The listing builds one solid part. Answer for the finished solid, in the listing's coordinates (mm). A direction names the side the tool comes from. Coordinates: 2 decimals unless noted, no trailing zeros. Order: outer loops, then holes, each group sorted by start corner. A loop starts at its lowest first (then second) coordinate and runs counter-clockwise, first axis right, second up. Notation, with made-up numbers: (57, 7) -> (77, 7) arc R18 ccw to (77, 22) -> close; hole circle Ø8 at (60, -33). An arc over 180 degrees is marked (long way). Write each question's results on one line, items separated by ' | '. Start each with the question number.
(1) Determine the mould class of faces 4 (the face through (-30, 0, 15)), 5 (the face through (39.724, -14.852, 3.204)), 6 (the face through (0, 0, 24.5)) for opening direction X: +X half, -X half, draft (parallel to the pull), parting line (faces both ways), or undercut.
(2) Straight lines are drawn through the part: L1, parallel to X at y = -13.5, z = 3; L2, parallel to X at y = 14.5, z = 5.75; L3, parallel to Y at x = -38.25, z = 4.75. For each, find the intervals that lie inside material, in ascending order.
(3) The part is cut by section D-D, the plane y = -13.5. Give the vertices of the cut face in (x, z), then the cut area to 3 significant figures.
(4) The part is cut by section A-A, the plane z = 3.5. Give the vertices of the cut face in (x, y), then the cut area to 3 significant figures.
(5) A tool of negligible diameter and unlimited length cuts with its end or side. For faces 1 (the face through (-36, 0, 6.5)), 2 (the face through (39.724, 12.148, 3.204)), 3 (the face through (30, 0, 15)), from which of +Z, -Z, +X, -X, +Y, -Y can it reach the whole face along a straight path? Write none if from no direction.
(6) The part is cut by section B-B, the plane y = -4. Give the vertices of the cut face in (x, z), then the cut area to 3 significant figures.
(7) Given pin 1 (2 mm diameter, centred on y = 12, z = 16, fed in from -X); pin 2 (5 mm diameter, centred on y = -6.5, z = 14, fed in from +X); pin 3 (3.5 mm diameter, centred on x = -34.5, y = 5, fed in from +Z); pin 4 (2.5 mm diameter, centred on x = -38.25, y = -13.5, fed in from +Z), each flat-ended and moving along its own axis, determine where each tip first touches the part or whether it passes through.
(8) The part is cut by section C-C, the plane x = 38.25. Give the vertices of the cut face in (y, z), then the cut area to 3 significant figures.
```python
from build123d import *

# Parameters (mm, degrees)
SKETCH_1_R      = 2
EXTRUDE_1_DEPTH = 6.5
SKETCH_2_W      = 60
SKETCH_2_H      = 40
EXTRUDE_2_DEPTH = 18


with BuildPart() as part:
    # ｽｹｯﾁ1 → ﾎﾞｽ - 押し出し1 (new body)
    with BuildSketch(Plane.XY):
        with BuildLine():
            Line((33, -20), (-33, -20))
            ThreePointArc((-33, -20), (-39.363961031, -17.363961031), (-42, -11))
            Line((-42, -11), (-42, 11))
            ThreePointArc((-42, 11), (-39.363961031, 17.363961031), (-33, 20))
            Line((-33, 20), (33, 20))
            ThreePointArc((33, 20), (39.363961031, 17.363961031), (42, 11))
            Line((42, 11), (42, -11))
            ThreePointArc((42, -11), (39.363961031, -17.363961031), (33, -20))
        make_face()
        with Locations(Location((-38.25, 13.5, 0), (0, 0, 180))):
            Circle(SKETCH_1_R, mode=Mode.SUBTRACT)
        with Locations(Location((38.25, 13.5, 0), (0, 0, 180))):
            Circle(SKETCH_1_R, mode=Mode.SUBTRACT)
        with Locations(Location((38.25, -13.5, 0), (0, 0, 180))):
            Circle(SKETCH_1_R, mode=Mode.SUBTRACT)
        with Locations(Location((-38.25, -13.5, 0), (0, 0, 180))):
            Circle(SKETCH_1_R, mode=Mode.SUBTRACT)
    extrude(amount=EXTRUDE_1_DEPTH)

    # ｽｹｯﾁ2 → ﾎﾞｽ - 押し出し2 (add)
    with BuildSketch(Plane.XY.offset(6.5)):
        Rectangle(SKETCH_2_W, SKETCH_2_H)
    extrude(amount=EXTRUDE_2_DEPTH)


solid = part.part
```
Established:
1) face 4: -X half | face 5: undercut | face 6: draft
2) L1: x = -41.65 to -40.25, -36.25 to 36.25, 40.25 to 41.65 | L2: x = -41.29 to -39.98, -36.52 to 36.52, 39.98 to 41.29 | L3: y = -18.31 to -15.5, -11.5 to 11.5, 15.5 to 18.31
3) outline: (-41.65, 0) -> (-40.25, 0) -> (-40.25, 6.5) -> (-41.65, 6.5) -> close; (-36.25, 0) -> (36.25, 0) -> (36.25, 6.5) -> (30, 6.5) -> (30, 24.5) -> (-30, 24.5) -> (-30, 6.5) -> (-36.25, 6.5) -> close; (40.25, 0) -> (41.65, 0) -> (41.65, 6.5) -> (40.25, 6.5) -> close | area: 1,570 mm^2
4) outline: (-42, -11) arc R9 ccw to (-33, -20) -> (33, -20) arc R9 ccw to (42, -11) -> (42, 11) arc R9 ccw to (33, 20) -> (-33, 20) arc R9 ccw to (-42, 11) -> close; hole circle Ø4 at (-38.25, -13.5); hole circle Ø4 at (-38.25, 13.5); hole circle Ø4 at (38.25, -13.5); hole circle Ø4 at (38.25, 13.5) | area: 3,240 mm^2
5) face 1: +Z, -X, +Y, -Y | face 2: +Z, -Z | face 3: +Z, +X, +Y, -Y
6) outline: (-42, 0) -> (42, 0) -> (42, 6.5) -> (30, 6.5) -> (30, 24.5) -> (-30, 24.5) -> (-30, 6.5) -> (-42, 6.5) -> close | area: 1,630 mm^2
7) pin 1: stops at x = -30 | pin 2: stops at x = 30 | pin 3: stops at z = 6.5 | pin 4: passes through
8) outline: (-18.31, 0) -> (-15.5, 0) -> (-15.5, 6.5) -> (-18.31, 6.5) -> close; (-11.5, 0) -> (11.5, 0) -> (11.5, 6.5) -> (-11.5, 6.5) -> close; (15.5, 0) -> (18.31, 0) -> (18.31, 6.5) -> (15.5, 6.5) -> close | area: 186 mm^2
